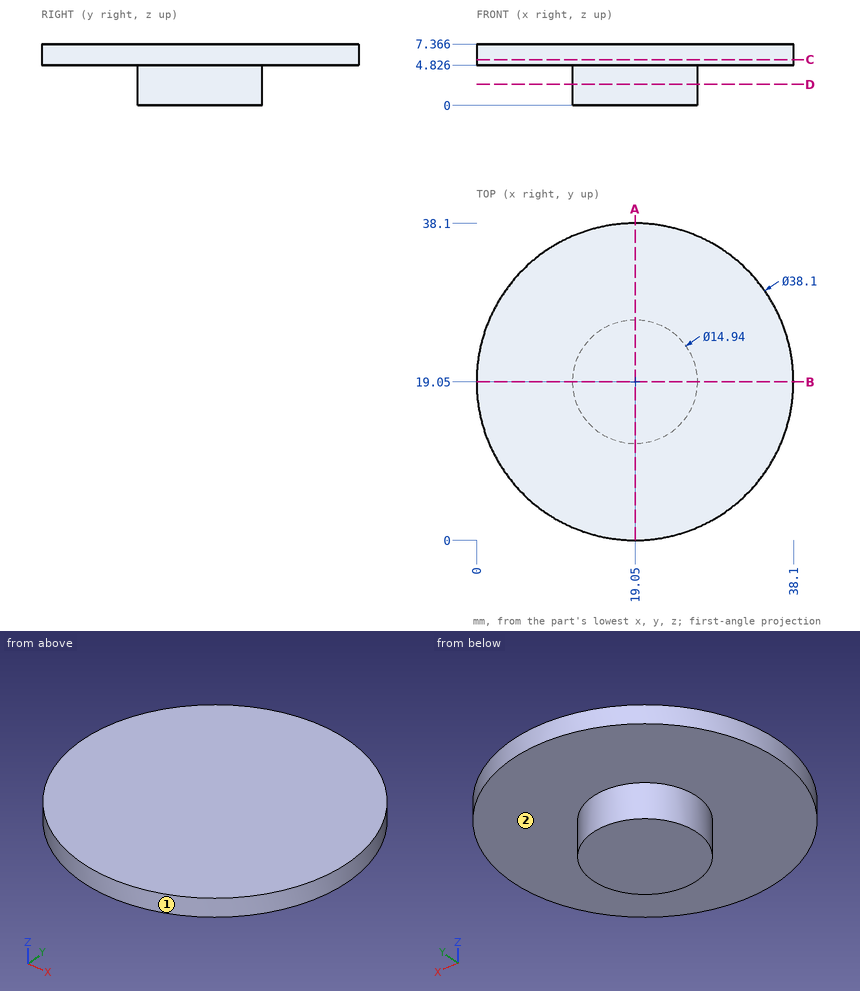
Design review of the part shown in the three views and the two pictorial views. Dimensions are in mm from the part's minimum x, y and z. A direction names the side the tool comes from. Give positions to 0.01 mm unless a question says otherwise; leave off trailing zeros. Write each loop counter-clockwise with the first axis right and the second up, starting at its lowest first coordinate (ties: lowest second). Pieces come first, ordered by that corner, then holes.
Item 1: Take a section at D-D (z = 2.5). Give the boundary of the cut face in (x, y).
Item 2: Machinability: for the marked faces 1 and 2, which of the approach directions +Z, -Z, +X, -X, +Y, -Y give a long, thin tool a straight path to every point of the face, cutting with its end or side? Answer none if there is none.
Item 3: Take a section at A-A (x = 19.05). Give the boundary of the cut face in (y, z), and give its area (3 significant figures).
Item 4: Wall thickness on probe 1 along Z at (x, y) = (3.5, 27.5); probe 2 along X at (y, z) = (31, 6); probe 3 along X at (y, z) = (18, 4): over which ranges is each line inside the solid? List them lowest first.
Item 5: Insertion check: P1, Ø1, axis at x = 5.5, y = 31, coming from the -Z side; P2, Ø6, axis at x = 18, y = 23.5, coming from the -Z side; P3, Ø4, axis at y = 29.5, z = 5.5, coming from the -X side; P4, Ø4, axis at x = 22.5, z = 4.5, coming from the -Y side. Each pin has a flat end and moves straight along its axis. Give the tip position at first contact, or say it passes through.
Item 6: Take a section at C-C (z = 5.5). Give the boundary of the cut face in (x, y).
Established:
1. outline: circle Ø14.94 at (19.05, 19.05)
2. face 1: +Z, -Z
2. face 2: -Z
3. outline: (0, 4.83) - (11.58, 4.83) - (11.58, 0) - (26.52, 0) - (26.52, 4.83) - (38.1, 4.83) - (38.1, 7.37) - (0, 7.37) - close
3. area: 169 mm2
4. probe 1: z = 4.83 to 7.37
4. probe 2: x = 4.21 to 33.89
4. probe 3: x = 11.65 to 26.45
5. P1: stops at z = 4.83
5. P2: stops at z = 0
5. P3: stops at x = 1.98
5. P4: stops at y = 0.06
6. outline: circle Ø38.1 at (19.05, 19.05)
